Model file for the job. Use its own axes, mm. A direction names the side the tool comes from. Coordinates: 2 decimals unless noted, no trailing zeros. Order: outer loops, then holes, each group sorted by start corner. A loop starts at its lowest first (then second) coordinate and runs counter-clockwise, first axis right, second up.
from build123d import *

# Parameters (mm, degrees)
F1_W     = 25.4
F1_H     = 25.4
F2_DEPTH = 101.6
F4_DEPTH = 25.4
F5_R     = 3.175
F6_R     = 6.7437
F7_DEPTH = 25.401


# Not quite as in the source:
# - a variable given as a bare number and used for a length is read in inches; the dataset says mm whatever the document's units were


with BuildPart() as f2:
    # F1 (on Top) → F2 (new body)
    with BuildSketch(Plane.XY):
        Rectangle(F1_W, F1_H)
        with BuildLine():
            ThreePointArc((-11.049, 7.874), (-10.1190640303, 10.1190640303), (-7.874, 11.049))
            Line((-7.874, 11.049), (7.874, 11.049))
            ThreePointArc((7.874, 11.049), (10.1190640303, 10.1190640303), (11.049, 7.874))
            Line((11.049, 7.874), (11.049, -7.874))
            ThreePointArc((11.049, -7.874), (10.1190640303, -10.1190640303), (7.874, -11.049))
            Line((7.874, -11.049), (-7.874, -11.049))
            ThreePointArc((-7.874, -11.049), (-10.1190640303, -10.1190640303), (-11.049, -7.874))
            Line((-11.049, -7.874), (-11.049, 7.874))
        make_face(mode=Mode.SUBTRACT)
    extrude(amount=F2_DEPTH)

    # F3 (on face) → F4 (cut)
    with BuildSketch(Plane.XZ.offset(12.7)):
        Polygon((12.7, 10.5210244843), (-12.7, 0), (12.7, 0), align=None)
        Polygon((12.7, 101.6), (-12.7, 101.6), (12.7, 91.0789755157), align=None)
    extrude(amount=-F4_DEPTH, mode=Mode.SUBTRACT)

    # F5
    f5_edges = [f2.edges().sort_by_distance(p)[0] for p in [
        (-12.7, 12.7, 50.8),
        (12.7, 12.7, 50.8),
        (-12.7, -12.7, 50.8),
        (12.7, -12.7, 50.8),
    ]]
    fillet(f5_edges, radius=F5_R)

    # F6 (on face) → F7 (cut, through all)
    with BuildSketch(Plane.XZ.offset(12.7)):
        with Locations((0, 50.8)):
            Circle(F6_R)
    extrude(amount=-F7_DEPTH, mode=Mode.SUBTRACT)


solid = f2.part
Q1. Probe line 1 (Y direction, x = -3.75, z = 73); line 2 (X direction, y = 9.5, z = 20). List the from-to ranges inside material, lowest first.
Established:
line 1: y = -12.7 to -11.05, 11.05 to 12.7
line 2: x = -12.7 to -10.6, 10.6 to 12.7
Q2. Which spindle directions (+Z, -Z, +X, -X, +Y, -Y) get a long thin tool onto all of the face, cutting with end or side? Do faces 1 (the face through (-0.178, -11.467, 96.413)), 2 (the face through (10.144, -10.094, 50.208)). Say none if no direction does.
Established:
face 1: +Z, +X, +Y, -Y
face 2: +Z, -Z
Q3. Cut at C-C, the plane x = 3.75. List the corners of the cut face in (y, z).
Established:
outline: (-12.7, 6.81) - (-11.05, 6.81) - (-11.05, 45.2) - (-12.7, 45.2) - close; (-12.7, 56.4) - (-11.05, 56.4) - (-11.05, 94.79) - (-12.7, 94.79) - close; (11.05, 6.81) - (12.7, 6.81) - (12.7, 45.2) - (11.05, 45.2) - close; (11.05, 56.4) - (12.7, 56.4) - (12.7, 94.79) - (11.05, 94.79) - close
Q4. Mould opens along Y. For faces 3 (the face through (-10.094, -10.144, 50.098)), 4 (the face through (-11.79, -11.75, 51.51)), 5 (the face through (-12.7, 0, 50)), 6 (the face through (-11.79, 11.75, 51.51)) say: pulls with the +Y half, pulls with the -Y half, needs draft (parallel to the pull), parting line crosses it, or undercut.
Established:
face 3: undercut
face 4: pulls with the -Y half
face 5: needs draft
face 6: pulls with the +Y half
Q5. Cut at B-B, the plane z = 50.8. List the corners of the cut face in (x, y) (3 decimals).
Established:
outline: (-12.7, -9.525) arc R3.175 ccw to (-9.525, -12.7) - (-6.744, -12.7) - (-6.744, -11.049) - (-7.874, -11.049) arc R3.175 cw to (-11.049, -7.874) - (-11.049, 7.874) arc R3.175 cw to (-7.874, 11.049) - (-6.744, 11.049) - (-6.744, 12.7) - (-9.525, 12.7) arc R3.175 ccw to (-12.7, 9.525) - close; (6.744, -12.7) - (9.525, -12.7) arc R3.175 ccw to (12.7, -9.525) - (12.7, 9.525) arc R3.175 ccw to (9.525, 12.7) - (6.744, 12.7) - (6.744, 11.049) - (7.874, 11.049) arc R3.175 cw to (11.049, 7.874) - (11.049, -7.874) arc R3.175 cw to (7.874, -11.049) - (6.744, -11.049) - close
Q6. Cut at A-A, the plane y = 1. List the corners of the cut face in (x, z), plus the area to 3 significant figures.
Established:
outline: (-12.7, 0) - (-11.05, 0.68) - (-11.05, 100.92) - (-12.7, 101.6) - close; (11.05, 9.84) - (12.7, 10.52) - (12.7, 91.08) - (11.05, 91.76) - close
area: 301 mm2
Q7. Drop flat-ended pins along their axis: P1, Ø6, axis at x = 0.5, y = 8.5, coming from the -Z side; P2, Ø8, axis at x = -7.5, y = 5.5, coming from the -Z side. Give the stop position or say it passes through.
Established:
P1: stops at z = 4.81
P2: stops at z = 0.5
